Print and shaded views of the part. All mm, measured from the part's lowest x, y and z. Round coordinates to 2 decimals unless told otherwise and drop trailing zeros. Loops run counter-clockwise (first coordinate to the right, second up) from the corner with the lowest first, then second, coordinate; pieces in that order, holes last. Notation, with made-up numbers: (13.25, 48.25) -> (41.25, 48.25) arc R22 cw to (41.25, 87.25) -> close; hole circle Ø1 at (-4.5, -7). An arc over 180 degrees is marked (long way). Use a Markdown table: item, result.
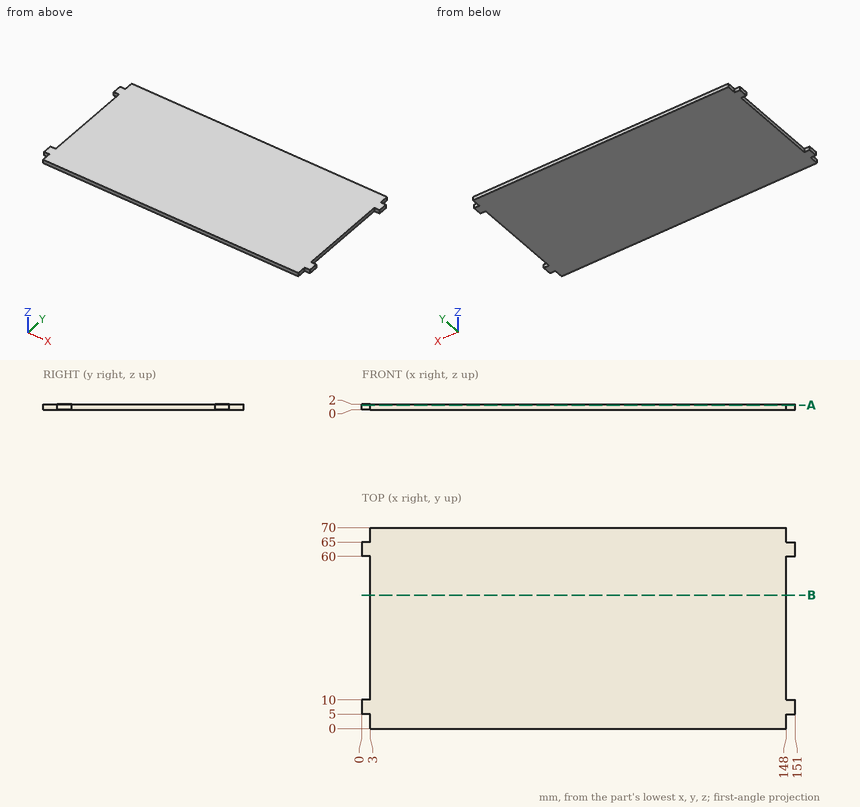
Q1. Flat gauge pins, fed straight in: pin 1 (1 mm diameter, centred on y = 68, z = 0.5, fed in from +X); pin 2 (0.6 mm diameter, centred on y = 37.5, z = 1, fed in from -X); pin 3 (0.6 mm diameter, centred on x = 1, z = 1, fed in from +Y). Where does each tip first touch, or does it go through?
Results list:
| item | result |
|---|---|
| pin 1 | stops at x = 148 |
| pin 2 | stops at x = 3 |
| pin 3 | stops at y = 65 |
Q2. Band-saw the part on A-A, the plane z = 1.65. Give the cut face in (x, y).
Results list:
| item | result |
|---|---|
| outline | (0, 5) -> (3, 5) -> (3, 0) -> (148, 0) -> (148, 5) -> (151, 5) -> (151, 10) -> (148, 10) -> (148, 60) -> (151, 60) -> (151, 65) -> (148, 65) -> (148, 70) -> (3, 70) -> (3, 65) -> (0, 65) -> (0, 60) -> (3, 60) -> (3, 10) -> (0, 10) -> close |
Q3. Band-saw the part on B-B, the plane y = 46.5. Give the cut face in (x, z).
Results list:
| item | result |
|---|---|
| outline | (3, 0) -> (148, 0) -> (148, 2) -> (3, 2) -> close |
Q4. Drill centre line: L1, parallel to X at y = 25, z = 1.45. Where is it in solid material? Low to high. Write a range as from..to.
Results list:
| item | result |
|---|---|
| L1 | x = 3..148 |
